For this review, take the finished solid that the model builds, in its own axes (mm). A direction names the side the tool comes from. Coordinates: 2 decimals unless noted, no trailing zeros. Loops run counter-clockwise (first coordinate to the right, second up) from the corner with the lowest first, then second, coordinate; pieces in that order, holes last. Notation, with made-up numbers: (53.5, -12) -> (109.5, -12) arc R14 cw to (109.5, -8) -> close; hole circle Ø6 at (52.25, 0.5). An arc over 180 degrees is marked (long way). One line per item, written item: value.
from build123d import *

# Parameters (mm, degrees)
F1_DEPTH        = 20
F2_R            = 5
F3_R            = 5
F4_R            = 10
F5_R            = 5
F6_R            = 5
F7_R            = 5
F8_R            = 5
F9_R            = 5
F10_R           = 1
F11_R           = 1
F12_T1_DEPTH    = 14.5857864376
F12_T3_DEPTH    = 44.2264973081
F12_T5_DEPTH    = 69.2264973081
F12_T7_DEPTH    = 18
F12_T9_DEPTH    = 10
F12_T14_DEPTH   = 1
F12_T20_DEPTH   = 1
F12_T24_ANGLE   = 90
F12_T26_ANGLE   = 90
F12_T28_ANGLE   = 60
F12_T30_ANGLE   = 60
F12_T32_ANGLE   = 90
F12_T34_ANGLE   = 90
F14_D           = 4
F14_CSINK_D     = 7
F14_CSINK_ANGLE = 90
F15_D           = 4
F15_CSINK_D     = 7
F15_CSINK_ANGLE = 90


# Not quite as in the source:
# - a fillet or chamfer that OpenCascade refuses, or shapes differently, is made with other operations: its cross-section is extruded or revolved along the edge and cut away or added


with BuildPart() as f1:
    # F0 (on Front) → F1 (new body)
    with BuildSketch(Plane.XZ):
        Polygon((42.1268583603, 53.609912917), (-27.1551739424, 13.609912917), (-27.1551739424, -46.390087083), (-2.1551739424, -46.390087083), (8.4514277754, -35.7834853652), (4.9158938694, -32.2479514593), (-4.1318040205, -41.2956493492), (-22.1551739424, -41.2956493492), (-22.1551739424, 10.7231615711), (44.6268583603, 49.2797858981), align=None)
    extrude(amount=F1_DEPTH)

    # F2
    f2_edges = [f1.edges().sort_by_distance(p)[0] for p in [
        (-22.155174, -10, -41.295649),
    ]]
    fillet(f2_edges, radius=F2_R)

    # F3
    f3_edges = [f1.edges().sort_by_distance(p)[0] for p in [
        (-4.131804, -10, -41.295649),
    ]]
    fillet(f3_edges, radius=F3_R)

    # F4
    f4_edges = [f1.edges().sort_by_distance(p)[0] for p in [
        (-27.155174, -10, -46.390087),
        (-27.155174, -10, 13.609913),
    ]]
    fillet(f4_edges, radius=F4_R)

    # F5
    f5_edges = [f1.edges().sort_by_distance(p)[0] for p in [
        (-22.155174, -10, 10.723162),
    ]]
    fillet(f5_edges, radius=F5_R)

    # F6
    f6_edges = [f1.edges().sort_by_distance(p)[0] for p in [
        (6.683661, 0, -34.015718),
    ]]
    fillet(f6_edges, radius=F6_R)

    # F7
    f7_edges = [f1.edges().sort_by_distance(p)[0] for p in [
        (6.683661, -20, -34.015718),
    ]]
    fillet(f7_edges, radius=F7_R)

    # F8
    f8_edges = [f1.edges().sort_by_distance(p)[0] for p in [
        (43.376858, -20, 51.444849),
    ]]
    fillet(f8_edges, radius=F8_R)

    # F9
    f9_edges = [f1.edges().sort_by_distance(p)[0] for p in [
        (43.376858, 0, 51.444849),
    ]]
    fillet(f9_edges, radius=F9_R)

    # F10
    f10_edges = [f1.edges().sort_by_distance(p)[0] for p in [
        (43.358594, -18.535534, 48.547553),
    ]]
    fillet(f10_edges, radius=F10_R)

    # F11
    f11_edges = [f1.edges().sort_by_distance(p)[0] for p in [
        (7.415894, -18.535534, -36.819019),
    ]]
    fillet(f11_edges, radius=F11_R)

    # F12: fillet of radius 1 on 14 edges, made by hand

    # F12_s2 → F12_t1 (cut)
    with BuildSketch(Plane.YZ.offset(-17.1551739424)):
        with BuildLine():
            ThreePointArc((0, -45.390087083), (-0.2928932188, -46.0971938642), (-1, -46.390087083))
            Line((-1, -46.390087083), (0, -46.390087083))
            Line((0, -46.390087083), (0, -45.390087083))
        make_face()
        with BuildLine():
            ThreePointArc((-19, -46.390087083), (-19.7071067812, -46.0971938642), (-20, -45.390087083))
            Line((-20, -45.390087083), (-20, -46.390087083))
            Line((-20, -46.390087083), (-19, -46.390087083))
        make_face()
    extrude(amount=F12_T1_DEPTH, mode=Mode.SUBTRACT)

    # F12_s4 → F12_t3 (cut)
    with BuildSketch(Plane.XY.offset(-36.390087083)):
        with BuildLine():
            ThreePointArc((-26.1551739424, 0), (-26.8622807236, -0.2928932188), (-27.1551739424, -1))
            Line((-27.1551739424, -1), (-27.1551739424, 0))
            Line((-27.1551739424, 0), (-26.1551739424, 0))
        make_face()
        with BuildLine():
            ThreePointArc((-27.1551739424, -19), (-26.8622807236, -19.7071067812), (-26.1551739424, -20))
            Line((-26.1551739424, -20), (-27.1551739424, -20))
            Line((-27.1551739424, -20), (-27.1551739424, -19))
        make_face()
    extrude(amount=F12_T3_DEPTH, mode=Mode.SUBTRACT)

    # F12_s6 → F12_t5 (cut)
    with BuildSketch(Plane(origin=(50.4787899917, 0, 29.1439429901), x_dir=(0, 1, 0), z_dir=(-0.8660254038, 0, -0.5))):
        with BuildLine():
            ThreePointArc((0, -24.3641173007), (-0.2928932188, -25.0712240818), (-1, -25.3641173007))
            Line((-1, -25.3641173007), (0, -25.3641173007))
            Line((0, -25.3641173007), (0, -24.3641173007))
        make_face()
        with BuildLine():
            ThreePointArc((-19, -25.3641173007), (-19.7071067812, -25.0712240818), (-20, -24.3641173007))
            Line((-20, -24.3641173007), (-20, -25.3641173007))
            Line((-20, -25.3641173007), (-19, -25.3641173007))
        make_face()
    extrude(amount=F12_T5_DEPTH, mode=Mode.SUBTRACT)

    # F12_s8 → F12_t7 (cut)
    with BuildSketch(Plane.XZ.offset(1)):
        with BuildLine():
            ThreePointArc((-2.5693875048, -46.390087083), (-2.1867040725, -46.3139666155), (-1.8622807236, -46.0971938642))
            Line((-1.8622807236, -46.0971938642), (-2.1551739424, -46.390087083))
            Line((-2.1551739424, -46.390087083), (-2.5693875048, -46.390087083))
        make_face()
    extrude(amount=F12_T7_DEPTH, mode=Mode.SUBTRACT)

    # F12_s10 → F12_t9 (cut)
    with BuildSketch(Plane.XZ.offset(5)):
        with BuildLine():
            ThreePointArc((41.2608329565, 53.109912917), (42.0196520016, 53.2098133395), (42.6268583603, 52.7438875132))
            Line((42.6268583603, 52.7438875132), (42.1268583603, 53.609912917))
            Line((42.1268583603, 53.609912917), (41.2608329565, 53.109912917))
        make_face()
    extrude(amount=F12_T9_DEPTH, mode=Mode.SUBTRACT)


with BuildPart() as f12_tool12:
    # F12_s13 → F12_t14 (new body)
    with BuildSketch(Plane.XZ.offset(19)):
        Polygon((-2.5693875048, -45.390087083), (-1.8622807236, -46.0971938642), (-2.1551739424, -46.390087083), (-2.5693875048, -46.390087083), align=None)
    extrude(amount=F12_T14_DEPTH)

    # F12_s15 → F12_t16 (revolve, cut)
    with BuildSketch(Plane(origin=(-2.5693875048, -19, -45.390087083), x_dir=(-0.3826834324, 0, 0.9238795325), z_dir=(0.9238795325, 0, 0.3826834324))):
        with BuildLine():
            ThreePointArc((0, -1), (1, 0), (0, 1))
            Line((0, 1), (0, -1))
        make_face()
    revolve(axis=Axis((-2.5693875048, -19, -45.390087083), (0, -1, 0)), mode=Mode.SUBTRACT)


with BuildPart() as f1_1:
    add(f1.part)

    # F12_t11: cut F12_tool12
    add(f12_tool12.part, mode=Mode.SUBTRACT)


with BuildPart() as f12_tool18:
    # F12_s19 → F12_t20 (new body)
    with BuildSketch(Plane.XZ.offset(1)):
        Polygon((-2.5693875048, -45.390087083), (-1.8622807236, -46.0971938642), (-2.1551739424, -46.390087083), (-2.5693875048, -46.390087083), align=None)
    extrude(amount=-F12_T20_DEPTH)

    # F12_s21 → F12_t22 (revolve, cut)
    with BuildSketch(Plane(origin=(-2.5693875048, -1, -45.390087083), x_dir=(-0.3826834324, 0, 0.9238795325), z_dir=(-0.9238795325, 0, -0.3826834324))):
        with BuildLine():
            ThreePointArc((0, -1), (1, 0), (0, 1))
            Line((0, 1), (0, -1))
        make_face()
    revolve(axis=Axis((-2.5693875048, -1, -45.390087083), (0, 1, 0)), mode=Mode.SUBTRACT)


with BuildPart() as f1_2:
    add(f1_1.part)

    # F12_t17: cut F12_tool18
    add(f12_tool18.part, mode=Mode.SUBTRACT)

    # F12_s23 → F12_t24 (revolve, cut)
    with BuildSketch(Plane.YZ.offset(-17.1551739424)):
        with BuildLine():
            ThreePointArc((-19, -46.390087083), (-19.7071067812, -46.0971938642), (-20, -45.390087083))
            Line((-20, -45.390087083), (-20, -46.390087083))
            Line((-20, -46.390087083), (-19, -46.390087083))
        make_face()
    revolve(axis=Axis((-17.1551739424, -20, -36.390087083), (0, 1, 0)), revolution_arc=F12_T24_ANGLE, mode=Mode.SUBTRACT)

    # F12_s25 → F12_t26 (revolve, cut)
    with BuildSketch(Plane.YZ.offset(-17.1551739424)):
        with BuildLine():
            ThreePointArc((0, -45.390087083), (-0.2928932188, -46.0971938642), (-1, -46.390087083))
            Line((-1, -46.390087083), (0, -46.390087083))
            Line((0, -46.390087083), (0, -45.390087083))
        make_face()
    revolve(axis=Axis((-17.1551739424, 0, -36.390087083), (0, 1, 0)), revolution_arc=F12_T26_ANGLE, mode=Mode.SUBTRACT)

    # F12_s27 → F12_t28 (revolve, cut)
    with BuildSketch(Plane(origin=(-9.4731152921, 0, -5.469305664), x_dir=(0, 1, 0), z_dir=(0.8660254038, 0, 0.5))):
        with BuildLine():
            ThreePointArc((0, 24.3641173007), (-0.2928932188, 25.0712240818), (-1, 25.3641173007))
            Line((-1, 25.3641173007), (0, 25.3641173007))
            Line((0, 25.3641173007), (0, 24.3641173007))
        make_face()
    revolve(axis=Axis((-17.1551739424, 0, 7.8364102251), (0, -1, 0)), revolution_arc=F12_T28_ANGLE, mode=Mode.SUBTRACT)

    # F12_s29 → F12_t30 (revolve, cut)
    with BuildSketch(Plane(origin=(-9.4731152921, 0, -5.469305664), x_dir=(0, 1, 0), z_dir=(0.8660254038, 0, 0.5))):
        with BuildLine():
            ThreePointArc((-19, 25.3641173007), (-19.7071067812, 25.0712240818), (-20, 24.3641173007))
            Line((-20, 24.3641173007), (-20, 25.3641173007))
            Line((-20, 25.3641173007), (-19, 25.3641173007))
        make_face()
    revolve(axis=Axis((-17.1551739424, -20, 7.8364102251), (0, -1, 0)), revolution_arc=F12_T30_ANGLE, mode=Mode.SUBTRACT)

    # F12_s31 → F12_t32 (revolve, cut)
    with BuildSketch(Plane.XZ.offset(5)):
        with BuildLine():
            ThreePointArc((41.2608329565, 53.109912917), (42.0196520016, 53.2098133395), (42.6268583603, 52.7438875132))
            Line((42.6268583603, 52.7438875132), (42.1268583603, 53.609912917))
            Line((42.1268583603, 53.609912917), (41.2608329565, 53.109912917))
        make_face()
    revolve(axis=Axis((37.7967313414, -5, 51.109912917), (-0.5, 0, 0.8660254038)), revolution_arc=F12_T32_ANGLE, mode=Mode.SUBTRACT)

    # F12_s33 → F12_t34 (revolve, cut)
    with BuildSketch(Plane(origin=(50.4787899917, 0, 29.1439429901), x_dir=(0, 1, 0), z_dir=(-0.8660254038, 0, -0.5))):
        with BuildLine():
            ThreePointArc((-19, -25.3641173007), (-19.7071067812, -25.0712240818), (-20, -24.3641173007))
            Line((-20, -24.3641173007), (-20, -25.3641173007))
            Line((-20, -25.3641173007), (-19, -25.3641173007))
        make_face()
    revolve(axis=Axis((37.7967313414, -15, 51.109912917), (-0.5, 0, 0.8660254038)), revolution_arc=F12_T34_ANGLE, mode=Mode.SUBTRACT)

    # F14 (through all)
    with Locations(Plane.YZ.offset(-22.1551739424)):
        with Locations((-13, -2.1635897749)):
            CounterSinkHole(F14_D / 2, F14_CSINK_D / 2, counter_sink_angle=F14_CSINK_ANGLE)

    # F15 (through all)
    with Locations(Plane.YZ.offset(-22.1551739424)):
        with Locations((-7, -16.2956493492)):
            CounterSinkHole(F15_D / 2, F15_CSINK_D / 2, counter_sink_angle=F15_CSINK_ANGLE)


solid = f1_2.part
1. Insertion check: pin 1 Ø4 at (x, y) = (21.5, -7.5) entering from +Z; pin 2 Ø10 at (x, y) = (23, -17.5) entering from -Z; pin 3 Ø1 at (x, y) = (-13, -4) entering from +Z; pin 4 Ø3 at (y, z) = (-7, -16.3) entering from -X. Each pin has a flat end and moves straight along its axis. Give the tip position at first contact, or say it passes through.
Return value:
pin 1: stops at z = 42.86
pin 2: stops at z = 33.91
pin 3: stops at z = 22.07
pin 4: passes through
2. Take a section at B-B, the plane z = -26. Give the boundary of the cut face in (x, y), and give its area (3 significant figures).
Return value:
outline: (-27.16, -19) arc R1 ccw to (-26.16, -20) -> (-23.16, -20) arc R1 ccw to (-22.16, -19) -> (-22.16, -1) arc R1 ccw to (-23.16, 0) -> (-26.16, 0) arc R1 ccw to (-27.16, -1) -> close
area: 99.1 mm2
3. Take a section at A-A, the plane y = -13. Give the boundary of the cut face in (x, z).
Return value:
outline: (-27.16, -36.39) arc R10 ccw to (-17.16, -46.39) -> (-2.57, -46.39) arc R1 ccw to (-1.86, -46.1) -> (7.74, -36.49) arc R1 ccw to (7.74, -35.08) -> (5.62, -32.96) arc R1 ccw to (4.21, -32.96) -> (-2.67, -39.83) arc R5 cw to (-6.2, -41.3) -> (-17.16, -41.3) arc R5 cw to (-22.16, -36.3) -> (-22.16, -5.66) -> (-23.66, -4.16) -> (-27.16, -4.16) -> close; (-27.16, -0.16) -> (-23.66, -0.16) -> (-22.16, 1.34) -> (-22.16, 7.84) arc R5 cw to (-19.66, 12.17) -> (43.76, 48.78) arc R1 ccw to (44.13, 50.15) -> (42.63, 52.74) arc R1 ccw to (41.26, 53.11) -> (-22.16, 16.5) arc R10 ccw to (-27.16, 7.84) -> close
4. The part is to be moulded in two halves that separate along Z. For faces 6 (the cylindrical face through (42.1, -1.5, 50.8)), 7 (the cylindrical face through (1.28, -19.7, -42.55)), 8 (the cylindrical face through (-21.467, -10.126, 10.368)), say which applies: pulls with the +Z half, pulls with the -Z half, needs draft (parallel to the pull), parting line crosses it, or undercut.
Return value:
face 6: pulls with the +Z half
face 7: pulls with the -Z half
face 8: undercut
5. To check wall thickness, follow probe 1 along X at (y, z) = (-6, -35); probe 2 along X at (y, z) = (-14, 2.5); probe 3 along Z at (x, y) = (-1, -6.5). State the ranges of each line that lie inside material, in increasing order. Write a range as from..to.
Return value:
probe 1: x = -27.16..-22.16, 2.16..7.67
probe 2: x = -27.16..-22.16
probe 3: z = -45.23..-38.16, 22.94..28.71
6. For faces 1 (the cylindrical face through (8.383, -19.699, 33.799)), 2 (the cylindrical face through (9.8, -0.3, 29.5)), 3 (the flat face through (-10, -10, -46.39)), 4 (the cylindrical face through (-4.315, -10.126, -40.925)), 5 (the flat face through (11.609, -9.874, 30.217)), list the 3-axis set-ups (+Z, -Z, +X, -X, +Y, -Y) from which the entire face can be reached by the end or side of a thin tool; tool diameter is ignored.
Return value:
face 1: +Z, -X, -Y
face 2: +X, +Y
face 3: -Z, +X, -X, +Y, -Y
face 4: +Y, -Y
face 5: +X, +Y, -Y
